The model under review builds one solid part; all positions refer to its coordinate system, in mm. Round coordinates to 2 decimals unless told otherwise and drop trailing zeros. Write each loop counter-clockwise with the first axis right and the second up, starting at its lowest first coordinate (ties: lowest second). Pieces come first, ordered by that corner, then holes.
Item 1: To check wall thickness, follow L1, parallel to Z at x = 0, y = -92; L2, parallel to Z at x = -1.25, y = -94.5; L3, parallel to Z at x = -0.25, y = -39.5. State the ranges of each line that lie inside material, in increasing order.
Item 2: Add section B-B (y = -64.5). Give the boundary of the cut face in (x, z).
Item 3: Add section A-A (y = -82.5). Give the boundary of the cut face in (x, z), plus the area to 3 significant figures.
Item 4: Clearance check with flat-ended pins moving along their axes: pin 1 Ø3 at (y, z) = (-65.5, 3.5) entering from -X; pin 2 Ø1.5 at (y, z) = (-88, 4) entering from -X; pin 3 Ø1 at (y, z) = (-56, -1) entering from -X. State where each tip first meets the part, or that it passes through.
Item 5: Draft analysis for pull direction X (two halves, no side actions). For faces 1 (the face through (0.585, -83.269, -2.636)), 2 (the face through (-0.1, -65.66, -0.46)), 3 (the face through (-1.08, -49.31, -4.88)), 4 (the face through (0, 0, 0)), state which applies: +X half, -X half, draft (parallel to the pull), parting line (faces both ways), or undercut.
```python
from build123d import *

# Parameters (mm, degrees)
F0_R     = 5
F1_DEPTH = 100
F2_SIZE  = 1
F4_D     = 5.4
F4_DEPTH = 33
F4_TIP   = 1.6223236714


with BuildPart() as f1:
    # F0 (on Front) → F1 (new body)
    with BuildSketch(Plane.XZ):
        Circle(F0_R)
    extrude(amount=F1_DEPTH)

    # F2
    f2_edges = [f1.edges().sort_by_distance(p)[0] for p in [
        (-5, -100, 0),
        (-5, 0, 0),
    ]]
    chamfer(f2_edges, length=F2_SIZE)

    # F4
    with Locations(Plane.XZ.offset(100)):
        with Locations((0, 0)):
            Hole(F4_D / 2, depth=F4_DEPTH)
            with Locations((0, 0, -(F4_DEPTH + F4_TIP / 2))):  # 118° drill point
                Cone(0, F4_D / 2, F4_TIP, mode=Mode.SUBTRACT)


solid = f1.part
```
Numbers:
1. L1: z = -5 to -2.7, 2.7 to 5
1. L2: z = -4.84 to -2.39, 2.39 to 4.84
1. L3: z = -4.99 to 4.99
2. outline: circle Ø10 at (0, 0)
3. outline: circle Ø10 at (0, 0); hole circle Ø5.4 at (0, 0)
3. area: 55.6 mm2
4. pin 1: stops at x = -4.58
4. pin 2: stops at x = -3.8
4. pin 3: stops at x = -4.97
5. face 1: undercut
5. face 2: undercut
5. face 3: parting line
5. face 4: draft
